Read the model definition and answer for the solid it produces. Units are mm, in the model's axes. Face numbers are marked on the shaded views. A direction names the side the tool comes from. Coordinates: 2 decimals unless noted, no trailing zeros. Loops run counter-clockwise (first coordinate to the right, second up) from the corner with the lowest first, then second, coordinate; pieces in that order, holes last. Notation, with made-up numbers: M -31,-2 L 14,-2 A30 ccw 14,26 Z; hole C -21,42 d8. An arc over 180 degrees is marked long. Put each result on its own line as item: value.
Autodesk Inventor part; units mm, degrees
ref_plane "YZ Plane" through (0, 0, 0) normal (1, 0, 0) x (0, 1, 0)
ref_plane "XZ Plane" through (0, 0, 0) normal (0, 1, 0) x (-1, 0, 0)
ref_plane "XY Plane" through (0, 0, 0) normal (0, 0, 1) x (1, 0, 0)
sketch "Sketch1" plane through (0, 0, 0) normal (0, 0, 1) x (1, 0, 0)
  circle A0 centre (0, 0) radius 19
  circle A1 centre (0, 0) radius 12.5
  dimension "d0" = 38
  dimension "d1" = 25
extrude "Extrusion1" add sketch "Sketch1" along normal blind 96 contours A1
extrude "Extrusion2" add sketch "Sketch1" along normal blind 12
sketch "Sketch2" plane through (0, 0, 0) normal (1, 0, 0) x (0, 1, 0)
  circle A0 centre (0, 84) radius 3
  line L0 (12.5, 96) -> (-12.5, 96)
  point P0 (0, 0)
  dimension "d6" = 6
  dimension "d7" = 12
extrude "Extrusion3" cut sketch "Sketch2" along normal through all both and the other way through all
properties part number "pin" material "Steel, Alloy"
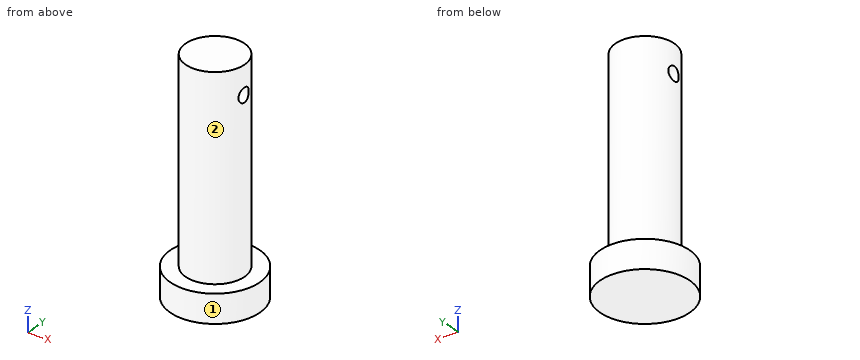
1) Find section C-C, the plane y = 8. Write down the section's boundary in (x, z).
Answer list:
outline: M -17.23,0 L 17.23,0 L 17.23,12 L 9.6,12 L 9.6,96 L -9.6,96 L -9.6,12 L -17.23,12 Z
2) Find section D-D, the plane z = 84. Write down the section's boundary in (x, y).
Answer list:
outline: M -12.13,-3 A12.5 ccw 12.13,-3 Z; M -12.13,3 L 12.13,3 A12.5 ccw Z
3) Find section B-B, the plane x = 0. Write down the section's boundary in (y, z), plus the area to 3 significant figures.
Answer list:
outline: M -19,0 L 19,0 L 19,12 L 12.5,12 L 12.5,96 L -12.5,96 L -12.5,12 L -19,12 Z; hole C 0,84 d6
area: 2,530 mm^2
4) Which of the six approach directions +Z, -Z, +X, -X, +Y, -Y give full straight-line access (tool end or side, diameter ignored) to the marked faces 1 and 2?
Answer list:
face 1: +Z, -Z
face 2: +Z
5) Find section A-A, the plane y = 0. Write down the section's boundary in (x, z), plus the area to 3 significant figures.
Answer list:
outline: M -19,0 L 19,0 L 19,12 L 12.5,12 L 12.5,81 L -12.5,81 L -12.5,12 L -19,12 Z; M -12.5,87 L 12.5,87 L 12.5,96 L -12.5,96 Z
area: 2,410 mm^2
6) Given pin 1 Ø4 at (y, z) = (6, 32.5) entering from -X; pin 2 Ø2 at (x, z) = (-3.5, 71) entering from +Y; pin 3 Ø5 at (y, z) = (0, 84) entering from +X; pin 4 Ø3 at (y, z) = (-4, 62) entering from -X, each flat-ended and moving along its own axis, determine where each tip first touches the part or whether it passes through.
Answer list:
pin 1: stops at x = -11.84
pin 2: stops at y = 12.25
pin 3: passes through
pin 4: stops at x = -12.25
7) Straight lines are drawn through the part: line 1 (Z direction, x = 0, y = 0); line 2 (Z direction, x = 1, y = -15); line 3 (Y direction, x = 5, z = 84). For each, find the intervals that lie inside material, in ascending order. Write a range as [from, to].
Answer list:
line 1: z = [0, 81], [87, 96]
line 2: z = [0, 12]
line 3: y = [-11.46, -3], [3, 11.46]
